Part model, mm, in its own coordinate system. Face numbers are marked on the shaded views. A direction names the side the tool comes from. Give positions to 0.01 mm unless a question says otherwise; leave off trailing zeros. Order: outer loops, then holes, each group sorted by start corner. A loop starts at its lowest first (then second) coordinate and runs counter-clockwise, first axis right, second up. Notation, with made-up numbers: M -16.5,-17 L 26.5,-17 A27 cw 26.5,-1 Z; hole C -34,20.5 d4. An arc over 180 degrees is marked long. Return JSON: item names as keys, results as strings.
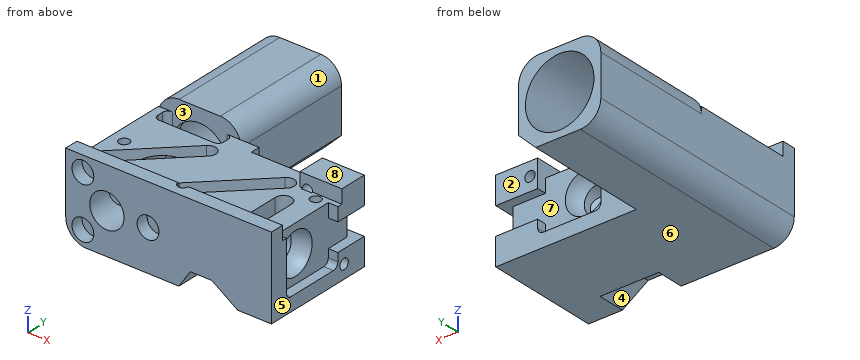
from build123d import *

# Parameters (mm, degrees)
SKETCH1_W                        = 15
SKETCH1_H                        = 6
MAIN_BODY_EXT_DEPTH              = 8.3
EMISSION_PATH_EXT_DEPTH          = 9
SKETCH3_R                        = 1.25
EMISSION_AND_GRIN_CUT_DEPTH      = 20.092931
SKETCH4_R                        = 1
DRUM_LENS_CUT_DEPTH              = 13
SKETCH41_R                       = 1
ADDTL_LIGHT_SOURCE_DEPTH         = 5
SKETCH5_W                        = 15
SKETCH5_H                        = 7.3
FILTERCOVER_CUT1_DEPTH           = 1
TOP_LED_SCREW_W                  = 3.06
TOP_LED_SCREW_H                  = 2
BOSS_EXTRUDE1_DEPTH              = 1
FILTERSET_CUT2_DEPTH             = 4
SKETCH10_R                       = 2.5
EMISSION_LENS_CUT_DEPTH          = 8.5
SKETCH15_R                       = 0.795
MAGNETS_CUT_DEPTH                = 0.9
SCREW_HOLES_CUT_DEPTH            = 20.507434
SCREW_HOLES_CUT_DEPTH_BACK       = 2.5
SKETCH18_R                       = 0.375
EXTERNAL_FILLET_1_R              = 1.5
VERTICAL_PATH_CUT_DEPTH          = 14.011149
VERTICAL_PATH_CUT_DEPTH_BACK     = 4
SKETCH28_R                       = 1.5
CUT_EXTRUDE_ORIGINAL_LIGHT_DEPTH = 0.7
CUT_EXTRUDE_ADDTL_LIGHT_DEPTH    = 0.7
SKETCH29_R                       = 0.375
SIDE_LED_SCREW_DEPTH             = 2.5
SKETCH32_W                       = 2
SKETCH32_H                       = 2.36
SIDE_WIRE_SLOT_CUT_DEPTH         = 0.7
SKETCH45_W                       = 2.36
SKETCH45_H                       = 2
TOP_LED_SLOT_DEPTH               = 0.7
CUT_EXTRUDE16_DEPTH              = 9
CUT_EXTRUDE17_REACH              = 13.945
SKETCH37_R                       = 2
SKETCH51_R                       = 0.375
TOP_LE_SCREW_DEPTH               = 2.1
CUT_EXTRUDE20_DEPTH              = 2


with BuildPart() as part:
    # Sketch1 → Main Body Ext (new body)
    with BuildSketch(Plane(origin=(0, 0, 0), x_dir=(1, 0, 0), z_dir=(0, 1, 0))):
        Rectangle(SKETCH1_W, SKETCH1_H)
    extrude(amount=MAIN_BODY_EXT_DEPTH)

    # Sketch8 → Emission Path Ext (add)
    with BuildSketch(Plane(origin=(0, 8.3, 0), x_dir=(1, 0, 0), z_dir=(0, 1, 0))):
        Polygon((-2.75, 3), (-1.5, 1.75), (-1.5, -3), (-7.5, -3), (-7.5, 3), align=None)
    extrude(amount=EMISSION_PATH_EXT_DEPTH)

    # Sketch3 → Emission and Grin Cut (cut, through all)
    with BuildSketch(Plane.XZ):
        with Locations(Location((-4.5, 0, 0), (0, 0, 270))):
            Circle(SKETCH3_R)
    extrude(amount=-EMISSION_AND_GRIN_CUT_DEPTH, mode=Mode.SUBTRACT)

    # Sketch4 → Drum Lens Cut (cut)
    with BuildSketch(Plane(origin=(7.5, 0, 0), x_dir=(0, 0, -1), z_dir=(1, 0, 0))):
        with Locations((0, 3)):
            Circle(SKETCH4_R)
    extrude(amount=-DRUM_LENS_CUT_DEPTH, mode=Mode.SUBTRACT)

    # Sketch41 → Addtl Light Source (cut)
    with BuildSketch(Plane(origin=(0, 8.3, 0), x_dir=(1, 0, 0), z_dir=(0, 1, 0))):
        with Locations(Location((1.5, 0, 0), (0, 0, 270))):
            Circle(SKETCH41_R)
    extrude(amount=-ADDTL_LIGHT_SOURCE_DEPTH, mode=Mode.SUBTRACT)

    # Sketch5 → FilterCover Cut1 (cut)
    with BuildSketch(Plane.XY.offset(3)):
        with Locations((0, 4.65)):
            Rectangle(SKETCH5_W, SKETCH5_H)
    extrude(amount=-FILTERCOVER_CUT1_DEPTH, mode=Mode.SUBTRACT)

    # Top-LED-Screw → Boss-Extrude1 (add)
    with BuildSketch(Plane.XY.offset(2)):
        with Locations((5.97, 7.3)):
            Rectangle(TOP_LED_SCREW_W, TOP_LED_SCREW_H)
    extrude(amount=BOSS_EXTRUDE1_DEPTH)

    # Sketch6 → FilterSet Cut2 (cut)
    with BuildSketch(Plane.XY.offset(2)):
        with BuildLine():
            Line((5.3, 4.5), (5.3, 1.8))
            ThreePointArc((5.3, 1.8), (5.7, 1.4), (5.3, 1))
            Line((5.3, 1), (4.1, 1))
            ThreePointArc((4.1, 1), (3.7, 1.4), (4.1, 1.8))
            Line((4.1, 1.8), (4.1, 4.5))
            ThreePointArc((4.1, 4.5), (4.7, 5.1), (5.3, 4.5))
        make_face()
        with BuildLine():
            Line((-6.9, 7.9), (-6.9, 7.5))
            ThreePointArc((-6.9, 7.5), (-6.782843, 7.217157), (-6.5, 7.1))
            Line((-6.5, 7.1), (-2.5, 7.1))
            ThreePointArc((-2.5, 7.1), (-2.217157, 7.217157), (-2.1, 7.5))
            Line((-2.1, 7.5), (-2.1, 7.9))
            ThreePointArc((-2.1, 7.9), (-2.217157, 8.182843), (-2.5, 8.3))
            Line((-2.5, 8.3), (-6.5, 8.3))
            ThreePointArc((-6.5, 8.3), (-6.782843, 8.182843), (-6.9, 7.9))
        make_face()
        with BuildLine():
            Line((-2.605887, 6.591169), (-6.848528, 2.348528))
            ThreePointArc((-6.848528, 2.348528), (-6.848528, 1.5), (-6, 1.5))
            Line((-6, 1.5), (-1.757359, 5.742641))
            ThreePointArc((-1.757359, 5.742641), (-1.757359, 6.591169), (-2.605887, 6.591169))
        make_face()
        with BuildLine():
            Line((3.112092, 6.591169), (-1.130548, 2.348528))
            ThreePointArc((-1.130548, 2.348528), (-1.130548, 1.5), (-0.28202, 1.5))
            Line((-0.28202, 1.5), (3.96062, 5.742641))
            ThreePointArc((3.96062, 5.742641), (3.96062, 6.591169), (3.112092, 6.591169))
        make_face()
    extrude(amount=-FILTERSET_CUT2_DEPTH, mode=Mode.SUBTRACT)

    # Sketch10 → Emission Lens Cut (cut)
    with BuildSketch(Plane(origin=(0, 17.3, 0), x_dir=(1, 0, 0), z_dir=(0, 1, 0))):
        with Locations(Location((-4.5, 0, 0), (0, 0, 270))):
            Circle(SKETCH10_R)
    extrude(amount=-EMISSION_LENS_CUT_DEPTH, mode=Mode.SUBTRACT)

    # Sketch15 → Magnets Cut (cut)
    with BuildSketch(Plane.XZ):
        with Locations(Location((-6.25, -1.875, 0), (0, 0, 270))):
            Circle(SKETCH15_R)
        with Locations(Location((-6.25, 1.875, 0), (0, 0, 270))):
            Circle(SKETCH15_R)
        with Locations(Location((-1.5, 0, 0), (0, 0, 270))):
            Circle(SKETCH15_R)
    extrude(amount=-MAGNETS_CUT_DEPTH, mode=Mode.SUBTRACT)

    # Sketch18 → Screw Holes Cut (cut, two sides: drawn at the far end of the back side and taken through both)
    with BuildSketch(Plane.XY.offset(2).offset(-SCREW_HOLES_CUT_DEPTH_BACK)):
        with Locations(Location((-6.5, 4, 0), (0, 0, 180))):
            Circle(SKETCH18_R)
        with Locations(Location((6, 5.8, 0), (0, 0, 180))):
            Circle(SKETCH18_R)
        with Locations((0.25, 1)):
            Circle(SKETCH18_R)
    extrude(amount=SCREW_HOLES_CUT_DEPTH + SCREW_HOLES_CUT_DEPTH_BACK, mode=Mode.SUBTRACT)

    # External Fillet 1
    # the kernel refuses this fillet: 1.5 mm, written as the material it takes off along each edge
    with BuildSketch(Plane(origin=(-7.5, -3.75, -3), x_dir=(1, 0, 0), z_dir=(0, 1, 0))) as external_fillet_1_piece_1:
        with BuildLine():
            CenterArc((EXTERNAL_FILLET_1_R, -EXTERNAL_FILLET_1_R), EXTERNAL_FILLET_1_R, 90, 90)
            Line((0, -EXTERNAL_FILLET_1_R), (0, 0))
            Line((0, 0), (EXTERNAL_FILLET_1_R, 0))
        make_face()
    extrude(amount=24.8, mode=Mode.SUBTRACT)
    with BuildSketch(Plane(origin=(-1.5, 8.3, 3), x_dir=(0, 0, -1), z_dir=(0, 1, 0))) as external_fillet_1_piece_2:
        with BuildLine():
            CenterArc((EXTERNAL_FILLET_1_R, EXTERNAL_FILLET_1_R), EXTERNAL_FILLET_1_R, 180, 90)
            Line((0, EXTERNAL_FILLET_1_R), (0, 0))
            Line((0, 0), (EXTERNAL_FILLET_1_R, 0))
        make_face()
    extrude(amount=12.75, mode=Mode.SUBTRACT)

    # Sketch28 → Vertical-Path-Cut (cut, two sides: drawn at the far end of the back side and taken through both)
    with BuildSketch(Plane(origin=(0, 7.1, 0), x_dir=(1, 0, 0), z_dir=(0, 1, 0)).offset(-VERTICAL_PATH_CUT_DEPTH_BACK)):
        with Locations(Location((-4.5, 0, 0), (0, 0, 180))):
            Circle(SKETCH28_R)
    extrude(amount=VERTICAL_PATH_CUT_DEPTH + VERTICAL_PATH_CUT_DEPTH_BACK, mode=Mode.SUBTRACT)

    # Sketch12 → Cut-Extrude Original Light (cut)
    with BuildSketch(Plane(origin=(7.5, 0, 0), x_dir=(0, 0, -1), z_dir=(1, 0, 0))):
        with BuildLine():
            Line((1.6, 5.94), (-1.6, 5.94))
            Line((-1.6, 5.94), (-2, 5.94))
            Line((-2, 5.94), (-2, 1.33))
            Line((-2, 1.33), (1.6, 1.33))
            ThreePointArc((1.6, 1.33), (1.882843, 1.447157), (2, 1.73))
            Line((2, 1.73), (2, 5.54))
            ThreePointArc((2, 5.54), (1.882843, 5.822843), (1.6, 5.94))
        make_face()
    extrude(amount=-CUT_EXTRUDE_ORIGINAL_LIGHT_DEPTH, mode=Mode.SUBTRACT)

    # Sketch44 → Cut-Extrude Addtl Light (cut)
    with BuildSketch(Plane(origin=(0, 8.3, 0), x_dir=(1, 0, 0), z_dir=(0, 1, 0))):
        with BuildLine():
            Line((-0.17, -2), (4.44, -2))
            Line((4.44, -2), (4.44, 1.6))
            ThreePointArc((4.44, 1.6), (4.322843, 1.882843), (4.04, 2))
            Line((4.04, 2), (0.23, 2))
            ThreePointArc((0.23, 2), (-0.052843, 1.882843), (-0.17, 1.6))
            Line((-0.17, 1.6), (-0.17, -2))
        make_face()
    extrude(amount=-CUT_EXTRUDE_ADDTL_LIGHT_DEPTH, mode=Mode.SUBTRACT)

    # Sketch29 → Side-LED-Screw (cut)
    with BuildSketch(Plane(origin=(7.5, 0, 0), x_dir=(0, 0, -1), z_dir=(1, 0, 0))):
        with Locations((2, 6.5)):
            Circle(SKETCH29_R)
    extrude(amount=-SIDE_LED_SCREW_DEPTH, mode=Mode.SUBTRACT)

    # Sketch32 → Side-Wire-Slot-Cut (cut)
    with BuildSketch(Plane(origin=(7.5, 0, 0), x_dir=(0, 0, -1), z_dir=(1, 0, 0))):
        with Locations((0, 7.12)):
            Rectangle(SKETCH32_W, SKETCH32_H)
    extrude(amount=-SIDE_WIRE_SLOT_CUT_DEPTH, mode=Mode.SUBTRACT)

    # Sketch45 → Top-LED-slot (cut)
    with BuildSketch(Plane(origin=(0, 8.3, 0), x_dir=(1, 0, 0), z_dir=(0, 1, 0))):
        with Locations((5.62, 0)):
            Rectangle(SKETCH45_W, SKETCH45_H)
    extrude(amount=-TOP_LED_SLOT_DEPTH, mode=Mode.SUBTRACT)

    # Sketch33 → Side-BallLens_Cut (revolve, cut)
    with BuildSketch(Plane.XY, mode=Mode.PRIVATE) as side_balllens_cut_sk:
        with BuildLine():
            Line((6.8, 3), (5.3, 3))
            ThreePointArc((5.3, 3), (5.73934, 4.06066), (6.8, 4.5))
            Line((6.8, 4.5), (6.8, 3))
        make_face()
    revolve(side_balllens_cut_sk.sketch.rotate(Axis((6.8, 3, 0), (-1, 0, 0)), 84.26086), axis=Axis((6.8, 3, 0), (-1, 0, 0)), mode=Mode.SUBTRACT)

    # Sketch47 → Top-BallLens_Cut (revolve, cut)
    with BuildSketch(Plane(origin=(1.5, 0, 0), x_dir=(0, 0, -1), z_dir=(1, 0, 0))):
        with BuildLine():
            Line((-1.5, 7.6), (0, 7.6))
            Line((0, 7.6), (0, 6.137287))
            ThreePointArc((0, 6.137287), (-1.04756, 6.563498), (-1.5, 7.6))
        make_face()
    revolve(axis=Axis((1.5, 7.6, 0), (0, -1, 0)), mode=Mode.SUBTRACT)

    # Sketch36 → Cut-Extrude16 (cut)
    with BuildSketch(Plane(origin=(0, 17.3, 0), x_dir=(1, 0, 0), z_dir=(0, 1, 0))):
        with BuildLine():
            Line((-7.5, -1.5), (-7.5, -3))
            Line((-7.5, -3), (-6, -3))
            ThreePointArc((-6, -3), (-7.06066, -2.56066), (-7.5, -1.5))
        make_face()
    extrude(amount=-CUT_EXTRUDE16_DEPTH, mode=Mode.SUBTRACT)

    # Sketch37 → Cut-Extrude17 (cut, up to next)
    with BuildSketch(Plane(origin=(0, 8.8, 0), x_dir=(1, 0, 0), z_dir=(0, 1, 0)), mode=Mode.PRIVATE) as cut_extrude17_sk1:
        with Locations(Location((-4.5, 0, 0), (0, 0, 180))):
            Circle(SKETCH37_R)
    cut_extrude17_tool1 = extrude(cut_extrude17_sk1.sketch, amount=-CUT_EXTRUDE17_REACH, mode=Mode.PRIVATE) & part.part
    add(cut_extrude17_tool1.solids().sort_by_distance((-4.5, 8.8, 0))[0], mode=Mode.SUBTRACT)

    # Sketch51 → Top-LE-Screw (cut)
    with BuildSketch(Plane(origin=(0, 8.3, 0), x_dir=(1, 0, 0), z_dir=(0, 1, 0))):
        with Locations(Location((5, -2, 0), (0, 0, 270))):
            Circle(SKETCH51_R)
    extrude(amount=-TOP_LE_SCREW_DEPTH, mode=Mode.SUBTRACT)

    # Notch → Cut-Extrude20 (cut)
    with BuildSketch(Plane.XZ):
        Polygon((3.151388, -1.7476), (1.584933, -1.7476), (1.584933, -3), (5.029987, -3), align=None)
        Polygon((1.584933, -3), (1.584933, -1.7476), (0.75, -3), align=None)
    extrude(amount=-CUT_EXTRUDE20_DEPTH, mode=Mode.SUBTRACT)


solid = part.part
Q1. Pin check, flat tips, straight feed: pin 1 (0.6 mm diameter, centred on x = -4, y = 7.5, fed in from +Z); pin 2 (1 mm diameter, centred on x = 4, y = 2, fed in from +Z); pin 3 (1.6 mm diameter, centred on x = 5.5, z = 2, fed in from +Y). Stop position of each tip, or through.
Established:
{"pin 1": "stops at z = -2", "pin 2": "stops at z = 2", "pin 3": "stops at y = 8.3"}
Q2. 3-axis set-ups, long thin cutter, end or side, ignore diameter. For the marked faces 1, 2, 3 and 4: which of +Z, -Z, +X, -X, +Y, -Y reach the whole face in a straight line?
Established:
{"face 1": "+Z, +X, +Y", "face 2": "+Z, -Z, +X, +Y", "face 3": "+Z", "face 4": "-Z, -Y"}
Q3. Probe line 1 along X through (y, z) = (12.75, 0); line 2 along Z through (x, y) = (-6, 13.5); line 3 along Y through (x, z) = (3.5, -0.85). List the from-to ranges inside material, lowest first.
Established:
{"line 1": "x = -7.5 to -7, -2 to -1.5", "line 2": "z = -3 to -2, 2 to 3", "line 3": "y = 0 to 2.47, 3.53 to 5.28, 6.77 to 7.6"}
Q4. Two-plate mould, pull along Z, no slides. Class the marked faces 5, 6, 7 and 8: +Z half, -Z half, draft (parallel to the pull), parting line (faces both ways), or undercut.
Established:
{"face 5": "draft", "face 6": "-Z half", "face 7": "undercut", "face 8": "+Z half"}
Q5. Band-saw the part on A-A (y = 11). Give the cut face in (x, z), then the cut area to 3 significant figures.
Established:
{"outline": "M -7.5,-1.5 A1.5 ccw -6,-3 L -2.75,-3 L -1.5,-1.75 L -1.5,1.5 A1.5 ccw -3,3 L -6,3 A1.5 ccw -7.5,1.5 Z; hole C -4.5,0 d5", "area": "14.1 mm²"}
